Check sheet for the modelled part. Datum: model origin and axes. Units: mm. A direction names the side the tool comes from. Round coordinates to 2 decimals unless told otherwise and drop trailing zeros. Order: outer loops, then holes, each group sorted by start corner. A loop starts at its lowest first (then second) coordinate and runs counter-clockwise, first axis right, second up. Notation, with made-up numbers: M 64.25,-10 L 85.25,-10 A21 cw 85.25,22 Z; hole C -32.75,2.5 d10. An arc over 180 degrees is marked long. One line per item, written item: value. Start each with the question number.
(1) Cross-section at B-B, the plane y = 38. Enter the section's corners in (x, z).
(2) Cross-section at C-C, the plane z = 64.5. Enter the section's corners in (x, y).
(3) Access from +Z, -Z, +X, -X, +Y, -Y to the whole of each face (thin tool, end or side, straight path). Record for faces 4 (the face through (9.229, 0.175, 92.743)), 5 (the face through (-11, -8, 46)), 6 (the face through (0, 12.5, 84)), 7 (the face through (-50, 0, 93)).
(4) Release check for a two-part mould opening along Z. For faces 1 (the face through (-59.86, -48.22, 65.83)), 2 (the face through (0, -12.5, 84)), 3 (the face through (-61.092, -3.252, 91.357)) record: released by +Z, released by -Z, zero draft, split by the parting line, or undercut.
(5) Thickness scan on L1, parallel to Z at x = -55.25, y = 0; L2, parallel to X at y = 0, z = 4.5; L3, parallel to Z at x = 0, y = -3. Record the ranges inside material, lowest first.
(6) Depth check by flat-ended pin: pin 1 Ø5 at (y, z) = (35.5, 37) entering from +X; pin 2 Ø1.5 at (x, y) = (36, 13.5) entering from +Z; pin 3 Ø2 at (y, z) = (2.5, 92.5) entering from -X. Enter the tip coordinate at first touch or a pass-through.
(7) Cross-section at D-D, the plane x = 15. Enter the section's corners in (y, z).
(8) Cross-section at A-A, the plane z = 106. Enter the section's corners in (x, y), and give its area (3 significant figures).
Autodesk Fusion 360 part; units mm, degrees
sketch "Sketch1" plane through (0, 0, 0) normal (0, 0, 1) x (1, 0, 0)
  line L0 (72.5, 68) -> (-72.5, 68)
  line L1 (-72.5, 68) -> (-72.5, -68)
  line L2 (-72.5, -68) -> (72.5, -68)
  line L3 (72.5, -68) -> (72.5, 68)
  line L4 (72.5, 68) -> (-72.5, -68) construction
  line L5 (-72.5, 68) -> (72.5, -68) construction
  dimension "d2" = 145
  dimension "d3" = 136
extrude "Extrude1" add sketch "Sketch1" along normal blind 136 makes body 1
sketch "Sketch2" plane through (0, -68, 0) normal (0, -1, 0) x (1, 0, 0)
  line L0 (-72.5, 0) -> (72.5, 0)
  line L1 (72.5, 0) -> (72.5, 136)
  line L2 (72.5, 136) -> (-72.5, 136)
  line L3 (-72.5, 136) -> (-72.5, 0)
  line L4 (-72.5, 136) -> (-50, 136)
  line L5 (-50, 136) -> (-50, 16)
  line L6 (-50, 16) -> (72.5, 16)
  line L7 (72.5, 0) -> (-72.5, 0)
  line L8 (72.5, 16) -> (72.5, 0)
  line L9 (-72.5, 0) -> (-72.5, 136)
  dimension "d6" = 136
  dimension "d7" = 16
extrude "Extrude2" cut sketch "Sketch2" against normal blind 290 contours L1 L2 L5 L6 bodies 1
sketch "Sketch3" plane through (-50, 0, 0) normal (1, 0, 0) x (0, 1, 0)
  line L0 (68, 16) -> (68, 136)
  line L1 (68, 136) -> (-68, 136)
  line L2 (-68, 136) -> (-68, 16)
  line L3 (-68, 16) -> (68, 16)
  line L4 (-68, 109.876) -> (68, 109.876) construction
  line L5 (0, 136) -> (0, 16) construction
  circle A0 centre (0, 109.876) radius 30
  circle A1 centre (0, 109.876) radius 15
  line L6 (-30, 109.876) -> (-68, 16)
  line L7 (30, 109.876) -> (68, 16)
  dimension "d10" = 60
  dimension "d11" = 30
extrude "Extrude3" cut sketch "Sketch3" against normal blind 50 contours L0 L1 A0 L7 | L1 L2 A0 L6 bodies 1
sketch "Sketch4" plane through (-50, 0, 0) normal (1, 0, 0) x (0, 1, 0)
  arc A0 (-14.7492, 136) -> (-30, 109.876) centre (0, 109.876) ccw
  line L0 (-30, 109.876) -> (-68, 16)
  line L1 (-68, 16) -> (68, 16)
  line L2 (68, 16) -> (30, 109.876)
  arc A1 (30, 109.876) -> (14.7492, 136) centre (0, 109.876) ccw
  line L3 (14.7492, 136) -> (-14.7492, 136)
  line L4 (-20, 106) -> (20, 106) construction
  circle A2 centre (0, 106) radius 15
  circle A3 centre (0, 106) radius 30
  point P0 (-68, 0)
  dimension "d14" = 106
  dimension "d15" = 30
  dimension "d16" = 60
extrude "Extrude4" cut sketch "Sketch4" against normal blind 50 contours A2 bodies 1
sketch "Sketch5" plane through (-50, 0, 0) normal (1, 0, 0) x (0, 1, 0)
  circle A0 centre (0, 106) radius 15
  arc A1 (-14.7492, 136) -> (-30, 109.876) centre (0, 109.876) ccw
  line L0 (-30, 109.876) -> (-68, 16)
  line L1 (-68, 16) -> (68, 16)
  line L2 (68, 16) -> (30, 109.876)
  arc A2 (30, 109.876) -> (14.7492, 136) centre (0, 109.876) ccw
  line L3 (14.7492, 136) -> (-14.7492, 136)
  circle A3 centre (0, 106) radius 30
  dimension "d19" = 60
extrude "Extrude5" cut sketch "Sketch5" against normal blind 120 contours A1 L0 L1 L2 A2 L3 bodies 1 makes body 2 at (-57.5, 29.8509, 103.013)
sketch "Sketch6" plane through (-50, 0, 0) normal (1, 0, 0) x (0, 1, 0)
  circle A0 centre (0, 106) radius 30
  circle A1 centre (0, 106) radius 15
  line L0 (68, 16) -> (27.8838, 117.0677)
  line L1 (0, 0) -> (0, 136) construction
  line L2 (68, 16) -> (27.8838, 117.0677)
  line L3 (-68, 16) -> (-27.8838, 117.0677)
  line L4 (-68, 16) -> (68, 16)
extrude "Extrude6" add sketch "Sketch6" against normal blind 20 contours A0 L0 L2 L3 L4 bodies 1 2
sketch "Sketch7" plane through (0, -68, 0) normal (0, -1, 0) x (1, 0, 0)
  line L0 (72.5, 16) -> (-50, 16)
  line L1 (-50, 16) -> (-70, 16)
  line L2 (-70, 16) -> (-72.5, 16)
  line L3 (-72.5, 16) -> (-72.5, 0)
  line L4 (-72.5, 0) -> (72.5, 0)
  line L5 (72.5, 0) -> (72.5, 16)
sketch "Sketch8" plane through (0, 0, 16) normal (0, 0, 1) x (-1, 0, 0)
  line L0 (50, -68) -> (50, 68)
  line L1 (50, 68) -> (-72.5, 68)
  line L2 (-72.5, 68) -> (-72.5, -68)
  line L3 (-72.5, -68) -> (50, -68)
  line L4 (50, 0) -> (-72.5, 0) construction
  circle A0 centre (-72.5, 0) radius 9
  circle A1 centre (-72.5, 0) radius 20
  dimension "d24" = 18
  dimension "d25" = 40
extrude "Extrude7" add sketch "Sketch8" along normal blind 25 contours L2 A0 A1 | L2 A0 A1 bodies 1
sketch "Sketch9" plane through (0, 0, 16) normal (0, 0, 1) x (-1, 0, 0)
  arc A0 (-72.5, -20) -> (-72.5, 20) centre (-72.5, 0) ccw
  line L0 (-72.5, -20) -> (-72.5, -68)
  line L1 (-72.5, -68) -> (50, -68)
  line L2 (50, -68) -> (50, 68)
  line L3 (50, 68) -> (-72.5, 68)
  line L4 (-72.5, 68) -> (-72.5, 20)
  line L5 (-72.5, -20) -> (50, -68)
  line L6 (50, -68) -> (-72.5, -68)
  line L7 (-72.5, -20) -> (-72.5, -68)
extrude "Extrude8" cut sketch "Sketch9" against normal blind 40 contours L0 L1 L5 L6 L7 bodies 1
sketch "Sketch10" plane through (0, 0, 16) normal (0, 0, 1) x (-1, 0, 0)
  line L0 (-72.5, -20) -> (50, -68)
  line L1 (50, -68) -> (50, 68)
  line L2 (50, 68) -> (-72.5, 68)
  line L3 (-72.5, 68) -> (-72.5, 20)
  arc A0 (-72.5, -20) -> (-72.5, 20) centre (-72.5, 0) ccw
  line L4 (-72.5, 20) -> (50, 68)
  line L5 (50, 68) -> (-72.5, 68)
  line L6 (-72.5, 68) -> (-72.5, 20)
extrude "Extrude9" cut sketch "Sketch10" against normal blind 50 contours L2 L3 L4 L5 L6 bodies 1
sketch "Sketch11" plane through (16.4434, -41.965, 0) normal (0.3648, -0.9311, 0) x (0.9311, 0.3648, 0)
  line L0 (-71.3621, 0) -> (60.2063, 0)
  line L1 (60.2063, 0) -> (60.2063, 16)
  line L2 (60.2063, 16) -> (-71.3621, 16)
  line L3 (-71.3621, 16) -> (-71.3621, 0)
extrude "Extrude10" cut 1 faces at (68.8622, 2.5078, 16) along direction (0, 0, -1) blind 40 on bodies 1 bodies 1
extrude "Extrude11" cut 1 faces at (56.2746, 1.4407, 41) along direction (0, 0, -1) blind 50 on bodies 1 bodies 1
sketch "Sketch12" plane through (0, 0, 16) normal (0, 0, 1) x (-1, 0, 0)
  line L0 (50, 68) -> (-72.5, 20)
  arc A0 (-72.5, -20) -> (-72.5, 20) centre (-72.5, 0) ccw
  line L1 (-72.5, -20) -> (50, -68)
  line L2 (50, -68) -> (50, 68)
sketch "Sketch13" plane through (0, 0, 0) normal (0, 0, -1) x (1, 0, 0)
  arc A0 (72.5, 20) -> (72.5, -20) centre (72.5, 0) ccw
  line L0 (72.5, 20) -> (-50, 68)
  line L1 (-50, 68) -> (-72.5, 68)
  line L2 (-72.5, 68) -> (-72.5, -68)
  line L3 (-72.5, -68) -> (-50, -68)
  line L4 (-50, -68) -> (72.5, -20)
  circle A1 centre (72.5, 0) radius 9
  circle A2 centre (72.5, 0) radius 20
  dimension "d37" = 18
  dimension "d38" = 40
extrude "Extrude12" add sketch "Sketch13" against normal blind 20 contours A0 A2 bodies 1
sketch "Sketch14" plane through (0, 0, 0) normal (0, 1, 0) x (1, 0, 0)
  line L0 (0, 0) -> (0, -61) construction
  line L1 (0, -61) -> (-75, -61) construction
  circle A0 centre (0, -75) radius 8
  circle A1 centre (0, -75) radius 20
  dimension "d43" = 61
  dimension "d44" = 75
  dimension "d45" = 16
  dimension "d46" = 40
extrude "Extrude13" add sketch "Sketch14" along normal blind 12.5 and the other way blind 12.5 separate body makes body 3
sketch "Sketch15" plane through (0, -68, 0) normal (0, -1, 0) x (1, 0, 0)
sketch "Sketch16" plane through (0, 0, 0) normal (0, 1, 0) x (1, 0, 0)
  line L0 (0, -95) -> (-50, -95)
  line L1 (-50, -95) -> (-50, -16)
  line L2 (-50, -16) -> (52.5, -16)
  line L3 (52.5, -16) -> (17.821, -84.078)
  circle A0 centre (0, -75) radius 20
extrude "Extrude14" add sketch "Sketch16" along normal blind 8 and the other way blind 8 contours L0 L1 L2 L3 A0 bodies 1 3
Values found:
1. outline: M -72.5,0 L 26.56,0 L 26.56,16 L -50,16 L -50,91.58 L -70,91.58 L -70,16 L -72.5,16 Z
2. outline: M -70,-48.75 L -50,-48.75 L -50,-8 L -17.02,-8 L -17.02,-12.5 L 17.02,-12.5 L 17.02,-8 L 27.79,-8 L 27.79,8 L 17.02,8 L 17.02,12.5 L -17.02,12.5 L -17.02,8 L -50,8 L -50,48.75 L -70,48.75 Z
3. face 4: none
3. face 5: -Y
3. face 6: +Z, +X, +Y
3. face 7: -X
4. face 1: released by +Z
4. face 2: zero draft
4. face 3: undercut
5. L1: 0 to 91, 121 to 136
5. L2: -72.5 to 63.5, 81.5 to 92.5
5. L3: 0 to 67, 83 to 95
6. pin 1: x = -50
6. pin 2: z = 16
6. pin 3: x = -50
7. outline: M -42.53,0 L 42.53,0 L 42.53,16 L 8,16 L 8,61.77 L 12.5,61.77 L 12.5,88.23 L -12.5,88.23 L -12.5,61.77 L -8,61.77 L -8,16 L -42.53,16 Z
8. outline: M -72.5,-30 L -70,-30 L -70,-32.28 L -50,-32.28 L -50,-15 L -72.5,-15 Z; M -72.5,15 L -50,15 L -50,32.28 L -70,32.28 L -70,30 L -72.5,30 Z
8. area: 766 mm^2
